```python
from build123d import *

# Parameters (mm, degrees)
SKETCH_1_W      = 6.2
SKETCH_1_H      = 1.3
SKETCH_1_W_2    = 1.3
SKETCH_1_H_2    = 6.2
SKETCH_1_W_3    = 10.5
SKETCH_1_H_3    = 10.5
SKETCH_1_R      = 3.4
EXTRUDE_2_DEPTH = 10


with BuildPart() as part:
    # 草图1 → 凸台-拉伸2 (new body)
    with BuildSketch(Plane(origin=(0, 0, 0), x_dir=(1, 0, 0), z_dir=(0, 1, 0))):
        with Locations((-7.3, -19.35)):
            Rectangle(SKETCH_1_W, SKETCH_1_H)
        with BuildLine():
            Line((-18.7, -10.4), (-20, -10.4))
            Line((-20, -10.4), (-20, -16.079155302))
            ThreePointArc((-20, -16.079155302), (-18.851611176, -18.851611176), (-16.079155302, -20))
            Line((-16.079155302, -20), (-10.4, -20))
            Line((-10.4, -20), (-10.4, -18.7))
            Line((-10.4, -18.7), (-10.4, -11.319238816))
            Line((-10.4, -11.319238816), (-10.4, -10.4))
            Line((-10.4, -10.4), (-11.319238816, -10.4))
            Line((-11.319238816, -10.4), (-18.7, -10.4))
        make_face()
        Polygon((-18.7, -15.2), (-18.7, -11.7), (-15.2, -11.7), (-11.7, -11.7), (-11.7, -15.2), (-11.7, -18.7), (-15.2, -18.7), (-18.7, -18.7), align=None, mode=Mode.SUBTRACT)
        with Locations((-19.35, -7.3)):
            Rectangle(SKETCH_1_W_2, SKETCH_1_H_2)
        with BuildLine():
            ThreePointArc((-15.2, -18.7), (-17.674873734, -17.674873734), (-18.7, -15.2))
            Line((-18.7, -15.2), (-18.7, -18.7))
            Line((-18.7, -18.7), (-15.2, -18.7))
        make_face()
        Polygon((-5.25, -5.25), (-5.25, -4.330761184), (-11.319238816, -10.4), (-10.4, -10.4), (-10.4, -11.319238816), (-4.330761184, -5.25), align=None)
        Rectangle(SKETCH_1_W_3, SKETCH_1_H_3)
        with Locations(Location((0, 0, 0), (0, 0, 270))):
            Circle(SKETCH_1_R, mode=Mode.SUBTRACT)
        Polygon((11.319238816, -10.4), (5.25, -4.330761184), (5.25, -5.25), (4.330761184, -5.25), (10.4, -11.319238816), (10.4, -10.4), align=None)
        Polygon((10.4, 11.319238816), (4.330761184, 5.25), (5.25, 5.25), (5.25, 4.330761184), (11.319238816, 10.4), (10.4, 10.4), align=None)
        Polygon((-4.330761184, 5.25), (-10.4, 11.319238816), (-10.4, 10.4), (-11.319238816, 10.4), (-5.25, 4.330761184), (-5.25, 5.25), align=None)
        with BuildLine():
            Line((18.7, -10.4), (11.319238816, -10.4))
            Line((11.319238816, -10.4), (10.4, -10.4))
            Line((10.4, -10.4), (10.4, -11.319238816))
            Line((10.4, -11.319238816), (10.4, -18.7))
            Line((10.4, -18.7), (10.4, -20))
            Line((10.4, -20), (16.079155302, -20))
            ThreePointArc((16.079155302, -20), (18.851611176, -18.851611176), (20, -16.079155302))
            Line((20, -16.079155302), (20, -10.4))
            Line((20, -10.4), (18.7, -10.4))
        make_face()
        Polygon((15.2, -11.7), (18.7, -11.7), (18.7, -15.2), (18.7, -18.7), (15.2, -18.7), (11.7, -18.7), (11.7, -15.2), (11.7, -11.7), align=None, mode=Mode.SUBTRACT)
        with BuildLine():
            Line((18.7, -18.7), (18.7, -15.2))
            ThreePointArc((18.7, -15.2), (17.674873734, -17.674873734), (15.2, -18.7))
            Line((15.2, -18.7), (18.7, -18.7))
        make_face()
        with BuildLine():
            Line((16.079155302, 20), (10.4, 20))
            Line((10.4, 20), (10.4, 18.7))
            Line((10.4, 18.7), (10.4, 11.319238816))
            Line((10.4, 11.319238816), (10.4, 10.4))
            Line((10.4, 10.4), (11.319238816, 10.4))
            Line((11.319238816, 10.4), (18.7, 10.4))
            Line((18.7, 10.4), (20, 10.4))
            Line((20, 10.4), (20, 16.079155302))
            ThreePointArc((20, 16.079155302), (18.851611176, 18.851611176), (16.079155302, 20))
        make_face()
        Polygon((15.2, 18.7), (18.7, 18.7), (18.7, 15.2), (18.7, 11.7), (15.2, 11.7), (11.7, 11.7), (11.7, 15.2), (11.7, 18.7), align=None, mode=Mode.SUBTRACT)
        with BuildLine():
            Line((18.7, 15.2), (18.7, 18.7))
            Line((18.7, 18.7), (15.2, 18.7))
            ThreePointArc((15.2, 18.7), (17.674873734, 17.674873734), (18.7, 15.2))
        make_face()
        with BuildLine():
            Line((-10.4, 20), (-16.079155302, 20))
            ThreePointArc((-16.079155302, 20), (-18.851611176, 18.851611176), (-20, 16.079155302))
            Line((-20, 16.079155302), (-20, 10.4))
            Line((-20, 10.4), (-18.7, 10.4))
            Line((-18.7, 10.4), (-11.319238816, 10.4))
            Line((-11.319238816, 10.4), (-10.4, 10.4))
            Line((-10.4, 10.4), (-10.4, 11.319238816))
            Line((-10.4, 11.319238816), (-10.4, 18.7))
            Line((-10.4, 18.7), (-10.4, 20))
        make_face()
        Polygon((-15.2, 11.7), (-18.7, 11.7), (-18.7, 15.2), (-18.7, 18.7), (-15.2, 18.7), (-11.7, 18.7), (-11.7, 15.2), (-11.7, 11.7), align=None, mode=Mode.SUBTRACT)
        with BuildLine():
            Line((-18.7, 18.7), (-18.7, 15.2))
            ThreePointArc((-18.7, 15.2), (-17.674873734, 17.674873734), (-15.2, 18.7))
            Line((-15.2, 18.7), (-18.7, 18.7))
        make_face()
        with Locations((-7.3, 19.35)):
            Rectangle(SKETCH_1_W, SKETCH_1_H)
        with Locations((7.3, 19.35)):
            Rectangle(SKETCH_1_W, SKETCH_1_H)
        with Locations((19.35, 7.3)):
            Rectangle(SKETCH_1_W_2, SKETCH_1_H_2)
        with Locations((-19.35, 7.3)):
            Rectangle(SKETCH_1_W_2, SKETCH_1_H_2)
        with Locations((19.35, -7.3)):
            Rectangle(SKETCH_1_W_2, SKETCH_1_H_2)
        with Locations((7.3, -19.35)):
            Rectangle(SKETCH_1_W, SKETCH_1_H)
    extrude(amount=EXTRUDE_2_DEPTH)


solid = part.part
```
Check sheet for the modelled part. Datum: model origin and axes. Units: mm. A direction names the side the tool comes from. Coordinates: 2 decimals unless noted, no trailing zeros. Write each loop counter-clockwise with the first axis right and the second up, starting at its lowest first coordinate (ties: lowest second). Pieces come first, ordered by that corner, then holes. Notation, with made-up numbers: M -19,18.5 L -6,18.5 A27 cw -6,57.5 Z; hole C 55.5,30.5 d6. An arc over 180 degrees is marked long. Write item = value, one per line. Start each with the question number.
1. Sectioned sample at B-B (x = 0). Record the cut outline in (y, z), then the cut area to 3 significant figures.
2. Tool access check on faces 1 (the flat face through (4.2, 5, 19)), 2 (the flat face through (-19, 5, 4.2)), 3 (the flat face through (-10, 5, -20)), 4 (the flat face through (15, 5, 11.7)). Record the directions out of +Z, -Z, +X, -X, +Y, -Y that give a thin tool (end or side, any length) a straight path to the whole face; none if there is none.
3. Sectioned sample at C-C (x = 14.5). Record the cut outline in (y, z), then the cut area to 3 significant figures.
4. Sectioned sample at A-A (z = 14.5). Record the cut outline in (x, y), then the cut area to 3 significant figures.
5. Go/stop test with flat-tipped pins: pin 1 (1 mm diameter, centred on y = 5.5, z = 19, fed in from -X); pin 2 (1.5 mm diameter, centred on x = -1, y = 7.5, fed in from -Z). Record where each tip stops, or that it passes through.
6. Thickness scan on probe 1 along X at (y, z) = (5.25, -14); probe 2 along X at (y, z) = (2, 0); probe 3 along X at (y, z) = (3.25, 6). Record the ranges inside material, lowest first.
7. Sectioned sample at D-D (z = 0). Record the cut outline in (x, y), then the cut area to 3 significant figures.
8. Mould release check, pull along X, two halves, no side actions. Record for faces 5 (the flat face through (15, 5, 10.4)), 6 (the flat face through (20, 5, 10)), 7 (the flat face through (-19, 5, -4.2)): pulls with the +X half, pulls with the -X half, needs draft (parallel to the pull), parting line crosses it, or undercut.
The answers:
q1.outline = M 0,-5.25 L 10,-5.25 L 10,-3.4 L 0,-3.4 Z; M 0,3.4 L 10,3.4 L 10,5.25 L 0,5.25 Z
q1.area = 37.0 mm²
q2.face_1 = +Z, +Y, -Y
q2.face_2 = -X, +Y, -Y
q2.face_3 = -Z, +X, -X, +Y, -Y
q2.face_4 = +Y, -Y
q3.outline = M 0,-20 L 10,-20 L 10,-18.7 L 0,-18.7 Z; M 0,-11.7 L 10,-11.7 L 10,-10.4 L 0,-10.4 Z; M 0,10.4 L 10,10.4 L 10,11.7 L 0,11.7 Z; M 0,18.7 L 10,18.7 L 10,20 L 0,20 Z
q3.area = 52.0 mm²
q4.outline = M -20,0 L -18.7,0 L -18.7,10 L -20,10 Z; M -11.7,0 L -10.4,0 L -10.4,10 L -11.7,10 Z; M 10.4,0 L 11.7,0 L 11.7,10 L 10.4,10 Z; M 18.7,0 L 20,0 L 20,10 L 18.7,10 Z
q4.area = 52.0 mm²
q5.pin_1 = -19.16
q5.pin_2 = -5.25
q6.probe_1 = -20 to -18.7, -11.7 to -10.4, 10.4 to 11.7, 18.7 to 20
q6.probe_2 = -5.25 to -3.4, 3.4 to 5.25
q6.probe_3 = -20 to -18.7, -6.92 to -5.08, 5.08 to 6.92, 18.7 to 20
q7.outline = M -5.25,0 L -3.4,0 L -3.4,10 L -5.25,10 Z; M 3.4,0 L 5.25,0 L 5.25,10 L 3.4,10 Z
q7.area = 37.0 mm²
q8.face_5 = undercut
q8.face_6 = pulls with the +X half
q8.face_7 = needs draft
